```python
from build123d import *

# Parameters (mm, degrees)
F0_R          = 14.2875
F0_R_2        = 12.319
F0_R_3        = 10.16
F1_DEPTH      = 25.4254
F0_R_4        = 17.4625
F2_DEPTH      = 12.7
F2_DEPTH_BACK = 0.0254
F3_START      = -25.4
F3_DEPTH      = 12.7
F4_START      = -33.02
F4_DEPTH      = 6.35


with BuildPart() as f1:
    # F0 (on Top) → F1 (new body)
    with BuildSketch(Plane.XY):
        Circle(F0_R)
        Circle(F0_R_2, mode=Mode.SUBTRACT)
        Circle(F0_R_2)
        Circle(F0_R_3, mode=Mode.SUBTRACT)
        Circle(F0_R_3)
    extrude(amount=-F1_DEPTH)

    # F0 (on Top) → F2 (join, two sides)
    with BuildSketch(Plane.XY) as f2_sk:
        Circle(F0_R_4)
        Circle(F0_R, mode=Mode.SUBTRACT)
    extrude(amount=-F2_DEPTH)
    extrude(f2_sk.sketch, amount=F2_DEPTH_BACK)

    # F0 (on Top) → F3 (join)
    with BuildSketch(Plane.XY.offset(F3_START)):
        Circle(F0_R_3)
    extrude(amount=-F3_DEPTH)

    # F0 (on Top) → F4 (join)
    with BuildSketch(Plane.XY.offset(F4_START)):
        Circle(F0_R_2)
        Circle(F0_R_3, mode=Mode.SUBTRACT)
    extrude(amount=-F4_DEPTH)


solid = f1.part
```
Work out the finished part from the listing and answer in its coordinate system (mm). A direction names the side the tool comes from. Round coordinates to 2 decimals unless told otherwise and drop trailing zeros. Order: outer loops, then holes, each group sorted by start corner. A loop starts at its lowest first (then second) coordinate and runs counter-clockwise, first axis right, second up.
Q1. Given pin 1 Ø4 at (x, y) = (1.5, 4.5) entering from +Z; pin 2 Ø6 at (x, z) = (6.5, -5) entering from -Y; pin 3 Ø6 at (x, y) = (-1, 2.5) entering from -Z; pin 4 Ø8.5 at (x, y) = (6.5, 7) entering from -Z, each flat-ended and moving along its own axis, determine where each tip first touches the part or whether it passes through.
Solution:
pin 1: stops at z = 0
pin 2: stops at y = -17.11
pin 3: stops at z = -38.1
pin 4: stops at z = -39.37
Q2. A tool of negligible diameter and unlimited length cuts with its end or side. For faces 1 (the cylindrical face through (-13.858, -10.626, -6.248)), 2 (the cylindrical face through (-1.323, 10.074, -38.726)), 3 (the flat face through (-10, -3, -25.425)), from which of +Z, -Z, +X, -X, +Y, -Y can it reach the whole face along a straight path? Write none if from no direction.
Solution:
face 1: +Z, -Z
face 2: -Z
face 3: none
Q3. Find the intervals of material crossed by line 1 along Z through (x, y) = (-10.5, 5); line 2 along Z through (x, y) = (-6.5, 4.5); line 3 along Z through (x, y) = (-12, -12.5), in increasing order.
Solution:
line 1: z = -39.37 to -33.02, -25.43 to 0
line 2: z = -38.1 to 0
line 3: z = -12.7 to 0.03
Q4. A cutting plane is placed at C-C, the plane z = -10. Determine the outline of the cut face in (x, y) (1 decimal).
Solution:
outline: circle Ø34.9 at (0, 0)
Q5. The mould has two halves that part along X. Classify faces 4 (the cylindrical face through (-1.323, 10.074, -29.17)), 5 (the flat face through (0, 0, -38.1)), 6 (the flat face through (-7, -13, 0.025)): pulls with the +X half, pulls with the -X half, needs draft (parallel to the pull), parting line crosses it, or undercut.
Solution:
face 4: parting line crosses it
face 5: undercut
face 6: needs draft
